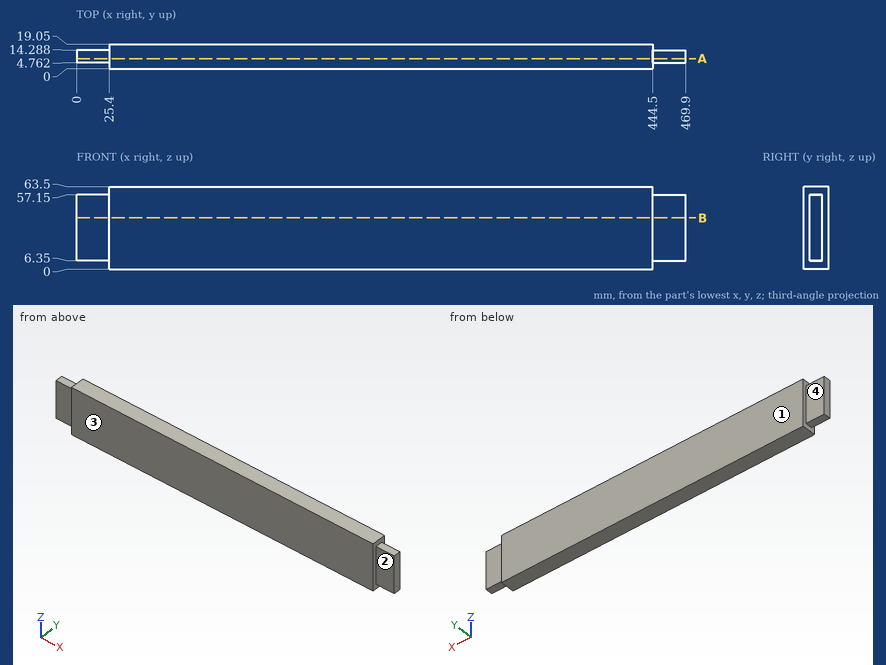
Source: three-view drawing plus pictorial views. Frame: mm from the lowest corner of the part. A direction names the side the tool comes from. Round coordinates to 2 decimals unless told otherwise and drop trailing zeros. Loops run counter-clockwise (first coordinate to the right, second up) from the corner with the lowest first, then second, coordinate; pieces in that order, holes last. Notation, with made-up numbers: M 2.25,-5 L 26.25,-5 A17 cw 26.25,3 Z; hole C -21,67.5 d10. An arc over 180 degrees is marked long. Put each result on its own line as item: value.
(1) Pull-direction query (Y, two-part tool) for the marked faces 1 and 2; classes: released by +Y, released by -Y, zero draft, split by the parting line, or undercut.
Solutions:
face 1: released by +Y
face 2: released by -Y
(2) Section A-A, the plane y = 7.75. Return loops of the section in (x, z), and give its area (3 significant figures).
Solutions:
outline: M 0,6.35 L 25.4,6.35 L 25.4,0 L 444.5,0 L 444.5,6.35 L 469.9,6.35 L 469.9,57.15 L 444.5,57.15 L 444.5,63.5 L 25.4,63.5 L 25.4,57.15 L 0,57.15 Z
area: 29,200 mm²
(3) First-contact query: pin 1 (10.5 mm diameter, centred on x = 13, y = 9.5, fed in from +Z); pin 2 (7.5 mm diameter, centred on x = 458, z = 39, fed in from -Y); pin 3 (10.5 mm diameter, centred on x = 455.5, y = 8, fed in from -Z). Flat tips, straight axial feed; report the tip coordinate or a pass-through.
Solutions:
pin 1: z = 57.15
pin 2: y = 4.76
pin 3: z = 6.35
(4) Ray query, line 1 (X direction, y = 17.5, z = 25.5); line 2 (Y direction, x = 447.5, z = 14). Return the intervals inside material, ascending. Write a range as [from, to].
Solutions:
line 1: [25.4, 444.5]
line 2: [4.76, 14.29]
(5) Section B-B, the plane z = 39.5. Return loops of the section in (x, y).
Solutions:
outline: M 0,4.76 L 25.4,4.76 L 25.4,0 L 444.5,0 L 444.5,4.76 L 469.9,4.76 L 469.9,14.29 L 444.5,14.29 L 444.5,19.05 L 25.4,19.05 L 25.4,14.29 L 0,14.29 Z
(6) Access query for the marked faces 3 and 4. Directions: +Z, -Z, +X, -X, +Y, -Y. A direction counts if a zero-diameter tool reaches every point of the face in a straight line with its end or side. Return the directions, or none.
Solutions:
face 3: +Z, -Z, +X, -X, -Y
face 4: +Z, -Z, -X, +Y
